Autodesk Inventor part; units mm, degrees
ref_plane "YZ Plane" through (0, 0, 0) normal (1, 0, 0) x (0, 1, 0)
ref_plane "XZ Plane" through (0, 0, 0) normal (0, 1, 0) x (-1, 0, 0)
ref_plane "XY Plane" through (0, 0, 0) normal (0, 0, 1) x (1, 0, 0)
sketch "Sketch1" plane through (0, 0, 0) normal (0, 1, 0) x (-1, 0, 0)
  line L0 (0, 0) -> (25, 0)
  line L1 (25, 0) -> (25, -25)
  line L2 (25, -25) -> (0, -25)
  line L3 (0, -25) -> (0, 0)
  line L4 (22, -22) -> (22, -3)
  line L5 (22, -3) -> (3, -3)
  line L6 (3, -3) -> (3, -22)
  line L7 (3, -22) -> (22, -22)
  dimension "d0" = 25
  dimension "d1" = 25
  dimension "d2" = 3
extrude "Extrusion1" add sketch "Sketch1" along normal blind 80
sketch "Sketch2" plane through (0, 0, 0) normal (1, 0, 0) x (0, 0, -1)
  line L0 (0, 0) -> (25, 0)
  line L1 (25, 0) -> (25, 80)
  line L2 (0, 80) -> (25, 80)
  line L3 (0, 0) -> (0, 80)
  line L4 (0, 0) -> (0, 80)
  line L5 (0, 80) -> (25, 55)
  line L6 (0, 80) -> (35.3553, 80) construction
  dimension "d5" = 45
extrude "Extrusion2" cut sketch "Sketch2" against normal blind 80 contours L2 L1 L5
sketch "Sketch3" plane through (-25, 0, 0) normal (0, 0, 1) x (1, 0, 0)
  line L0 (3, 0) -> (3, 77)
  line L1 (0, 0) -> (25, 0)
  line L2 (25, 0) -> (25, 80)
  line L3 (0, 80) -> (25, 80)
  line L4 (0, 0) -> (0, 80)
  line L5 (25, 0) -> (0, 0)
  line L6 (0, 25) -> (25, 0)
  dimension "d8" = 45
extrude "Extrusion3" cut sketch "Sketch3" against normal blind 44.75 contours L1 L4 L6 L0 | L0 L6 L1
properties part number "P404" material "Aluminum 6061"
Read the model definition and answer for the solid it produces. Units are mm, in the model's axes. A direction names the side the tool comes from. Coordinates: 2 decimals unless noted, no trailing zeros. Loops run counter-clockwise (first coordinate to the right, second up) from the corner with the lowest first, then second, coordinate; pieces in that order, holes last.
Q1. The part is cut by section D-D on y = 39.5. Write down the section's boundary in (x, z).
Q2. The part is cut by section B-B on x = -13.25. Write down the section's boundary in (y, z), and give its area (4 significant figures).
Q3. The part is cut by section C-C on y = 67. Write down the section's boundary in (x, z).
Q4. Consider probe 1 along X at (y, z) = (38.5, -16.75); probe 2 along X at (y, z) = (14, -9.5). Determine where each line is inside the solid, lowest interval first.
Q5. The mould has two halves that part along Z. Classify faces 3 (the face through (0, 31, -13)), 4 (the face through (-3, 31, -12)), 5 (the face through (-12, 48, 0)): +Z half, -Z half, draft (parallel to the pull), parting line (faces both ways), or undercut.
Q6. The part is cut by section A-A on z = -20.25. Write down the section's boundary in (x, y), and give its area (4 significant figures).
Q7. Which of the six approach directions +Z, -Z, +X, -X, +Y, -Y give full straight-line access (tool end or side, diameter ignored) to faces 1 (the face through (-12, 36, -22)), 2 (the face through (-13, 33, -25))?
Results below:
1. outline: (-25, -25) - (0, -25) - (0, 0) - (-25, 0) - close; hole (-22, -22) - (-3, -22) - (-3, -3) - (-22, -3) - close
2. outline: (13.25, -25) - (55, -25) - (58, -22) - (13.25, -22) - close; (13.25, -3) - (77, -3) - (80, 0) - (13.25, 0) - close
2. area: 325.5 mm2
3. outline: (-25, -13) - (-22, -13) - (-22, -3) - (-3, -3) - (-3, -13) - (0, -13) - (0, 0) - (-25, 0) - close
4. probe 1: x = -25 to -22, -3 to 0
4. probe 2: x = -3 to 0
5. face 3: draft
5. face 4: undercut
5. face 5: +Z half
6. outline: (-25, 25) - (-22, 22) - (-22, 59.75) - (-25, 59.75) - close; (-3, 3) - (0, 0) - (0, 59.75) - (-3, 59.75) - close
6. area: 283.5 mm2
7. face 1: +Y, -Y
7. face 2: -Z, +X, -X, +Y, -Y
